```python
from build123d import *

# Parameters (mm, degrees)
SKETCH_1_W             = 150
SKETCH_1_H             = 245
SM_BASE_FLANGE_1_DEPTH = 20
CHAMFER_1_SIZE         = 16
CHAMFER_1_SIZE2        = 11.203320611
CHAMFER_2_SIZE         = 16
CHAMFER_2_SIZE2        = 11.203320611


# Sheet-metal steps are written as plain solids
with BuildPart() as part:
    # Sketch 1 → 基体-法兰1 (new body)
    with BuildSketch(Plane.XY):
        Rectangle(SKETCH_1_W, SKETCH_1_H)
    extrude(amount=-SM_BASE_FLANGE_1_DEPTH)

    # 倒角1
    chamfer_1_edges = [part.edges().sort_by_distance(p)[0] for p in [
        (0, 122.5, -20),
    ]]
    chamfer_1_side = [part.faces().sort_by_distance(p)[0] for p in [
        (0, 122.5, -10),
    ]]
    chamfer(chamfer_1_edges, length=CHAMFER_1_SIZE, length2=CHAMFER_1_SIZE2, reference=chamfer_1_side[0])

    # 倒角2
    chamfer_2_edges = [part.edges().sort_by_distance(p)[0] for p in [
        (0, -122.5, -20),
    ]]
    chamfer_2_side = [part.faces().sort_by_distance(p)[0] for p in [
        (0, -122.5, -10),
    ]]
    chamfer(chamfer_2_edges, length=CHAMFER_2_SIZE, length2=CHAMFER_2_SIZE2, reference=chamfer_2_side[0])


solid = part.part
```
Here's how the part is built. I have some questions about the finished solid (model axes, mm). Coordinates: 2 decimals unless noted, no trailing zeros. Order: outer loops, then holes, each group sorted by start corner. A loop starts at its lowest first (then second) coordinate and runs counter-clockwise, first axis right, second up. Notation, with made-up numbers: M 13,71.25 L 25,71.25 A4 cw 25,78.25 Z; hole C -9,6 d6. An arc over 180 degrees is marked long. Answer as a JSON object with one key per item and string values. Group by question number.
(1) I need wall thicknesses on probe 1 along Y at (x, z) = (48.5, -19); probe 2 along Y at (x, z) = (15.5, -17). Which ranges of each line are inside material? Lowest first, please.
(2) For pin 1 (6 mm diameter, centred on x = 6, z = -11, fed in from -Y); pin 2 (6 mm diameter, centred on x = 23.5, z = -11.5, fed in from +Y); pin 3 (3 mm diameter, centred on x = 57.5, z = -12.5, fed in from -Y), each with a flat end and sliding along its axis, tell me the tip position at first contact or that it passes through.
(3) Suppose I cut it at A-A, the plane x = 12.5. Please give me the cut outline in (y, z).
(4) Suppose I cut it at B-B, the plane z = -8.25. Please give me the cut outline in (x, y).
Values found:
{
 "1": {"probe 1": "y = -112 to 112", "probe 2": "y = -113.4 to 113.4"},
 "2": {"pin 1": "stops at y = -119.7", "pin 2": "stops at y = 119.35", "pin 3": "stops at y = -117.6"},
 "3": {"outline": "M -122.5,-4 L -111.3,-20 L 111.3,-20 L 122.5,-4 L 122.5,0 L -122.5,0 Z"},
 "4": {"outline": "M -75,-119.52 L 75,-119.52 L 75,119.52 L -75,119.52 Z"}
}
